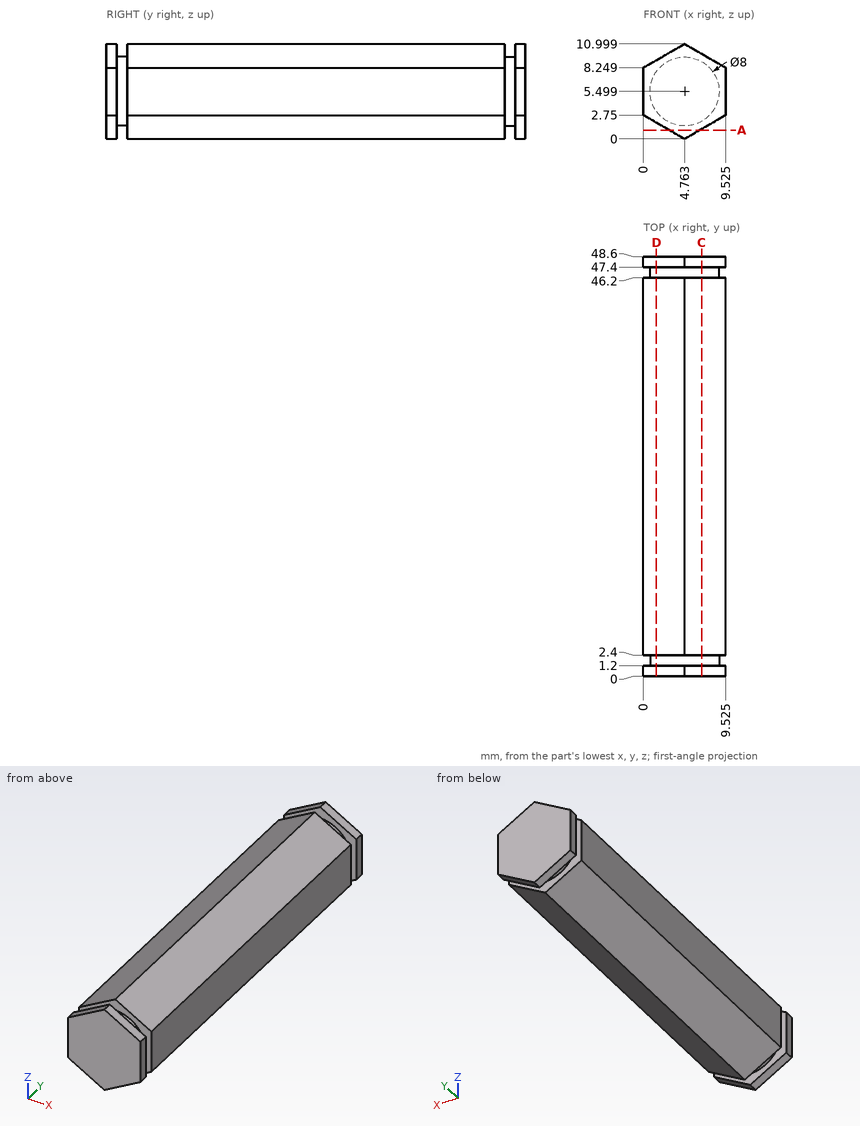
Print and shaded views of the part. All mm, measured from the part's lowest x, y and z. Give positions to 0.01 mm unless a question says otherwise; leave off trailing zeros. Loops run counter-clockwise (first coordinate to the right, second up) from the corner with the lowest first, then second, coordinate; pieces in that order, holes last. Notation, with made-up numbers: (2.25, -6.5) -> (21.25, -6.5) arc R18 cw to (21.25, 8.5) -> close; hole circle Ø7 at (-28, 49). An arc over 180 degrees is marked (long way). Use a Markdown table: item, result.
1. Slice it at A-A (z = 1). List the corners of the cut face in (x, y) (1 decimal).
Check result:
| item | result |
|---|---|
| outline | (3, 0) -> (6.5, 0) -> (6.5, 1.2) -> (3, 1.2) -> close; (3, 2.4) -> (6.5, 2.4) -> (6.5, 46.2) -> (3, 46.2) -> close; (3, 47.4) -> (6.5, 47.4) -> (6.5, 48.6) -> (3, 48.6) -> close |
2. Slice it at C-C (x = 6.75). List the corners of the cut face in (y, z).
Check result:
| item | result |
|---|---|
| outline | (0, 1.15) -> (1.2, 1.15) -> (1.2, 2.03) -> (2.4, 2.03) -> (2.4, 1.15) -> (46.2, 1.15) -> (46.2, 2.03) -> (47.4, 2.03) -> (47.4, 1.15) -> (48.6, 1.15) -> (48.6, 9.85) -> (47.4, 9.85) -> (47.4, 8.97) -> (46.2, 8.97) -> (46.2, 9.85) -> (2.4, 9.85) -> (2.4, 8.97) -> (1.2, 8.97) -> (1.2, 9.85) -> (0, 9.85) -> close |
3. Wall check: L1, parallel to Y at x = 7.5, z = 1.75; L2, parallel to X at y = 38, z = 8.5 (1 decimal); L3, parallel to Z at x = 6.5, y = 27.5 (1 decimal). Give the ranges that are in metal, low to high. Write a range as [from, to].
Check result:
| item | result |
|---|---|
| L1 | y = [0, 1.2], [2.4, 46.2], [47.4, 48.6] |
| L2 | x = [0.4, 9.1] |
| L3 | z = [1, 10] |
4. Flat gauge pin, fed straight in: pin 1 (4 mm diameter, centred on x = 4.5, y = 38.5, fed in from +Z). Where does the tip first touch, or does it go through?
Check result:
| item | result |
|---|---|
| pin 1 | stops at z = 11 |
5. Slice it at D-D (x = 1.5). List the corners of the cut face in (y, z) (1 decimal).
Check result:
| item | result |
|---|---|
| outline | (0, 1.9) -> (1.2, 1.9) -> (1.2, 3.2) -> (2.4, 3.2) -> (2.4, 1.9) -> (46.2, 1.9) -> (46.2, 3.2) -> (47.4, 3.2) -> (47.4, 1.9) -> (48.6, 1.9) -> (48.6, 9.1) -> (47.4, 9.1) -> (47.4, 7.8) -> (46.2, 7.8) -> (46.2, 9.1) -> (2.4, 9.1) -> (2.4, 7.8) -> (1.2, 7.8) -> (1.2, 9.1) -> (0, 9.1) -> close |
